from build123d import *

# Parameters (mm, degrees)
F0_W       = 2.5
F0_H       = 32
F0_H_2     = 52
F1_DEPTH   = 5
F2_DEPTH   = 20
F3_W       = 15
F3_H       = 15
F3_R       = 2.5
F4_W       = 15
F4_H       = 15
F4_R       = 2.5
F5_DEPTH   = 5
F6_SIZE2   = 2.14473742
F6_SIZE    = 2
F7_SIZE2   = 2.14473742
F7_SIZE    = 2
F8_SIZE2   = 2.14473742
F8_SIZE    = 2
F8_2_SIZE2 = 2.14473742
F8_2_SIZE  = 2


with BuildPart() as f1:
    # F0 (on Top) → F1 (new body)
    with BuildSketch(Plane.XY):
        Polygon((61.6508859247, 52.6726719439), (-55.3491140753, 52.6726719439), (-55.3491140753, 37.6726719439), (-52.8491140753, 37.6726719439), (-52.8491140753, 50.1726719439), (59.1508859247, 50.1726719439), (59.1508859247, 27.6726719439), (61.6508859247, 27.6726719439), align=None)
        Polygon((-52.8491140753, 50.1726719439), (-52.8491140753, 37.6726719439), (-52.8491140753, -14.3273280561), (-52.8491140753, -26.8273280561), (59.1508859247, -26.8273280561), (59.1508859247, -4.3273280561), (59.1508859247, 27.6726719439), (59.1508859247, 50.1726719439), align=None)
        with Locations((60.4008859247, 11.6726719439)):
            Rectangle(F0_W, F0_H)
        Polygon((-52.8491140753, -14.3273280561), (-55.3491140753, -14.3273280561), (-55.3491140753, -29.3273280561), (61.6508859247, -29.3273280561), (61.6508859247, -4.3273280561), (59.1508859247, -4.3273280561), (59.1508859247, -26.8273280561), (-52.8491140753, -26.8273280561), align=None)
        with Locations((-54.0991140753, 11.6726719439)):
            Rectangle(F0_W, F0_H_2)
    extrude(amount=-F1_DEPTH)

    # F0 (on Top) → F2 (join)
    with BuildSketch(Plane.XY):
        Polygon((61.6508859247, 52.6726719439), (-55.3491140753, 52.6726719439), (-55.3491140753, 37.6726719439), (-52.8491140753, 37.6726719439), (-52.8491140753, 50.1726719439), (59.1508859247, 50.1726719439), (59.1508859247, 27.6726719439), (61.6508859247, 27.6726719439), align=None)
        Polygon((-52.8491140753, -14.3273280561), (-55.3491140753, -14.3273280561), (-55.3491140753, -29.3273280561), (61.6508859247, -29.3273280561), (61.6508859247, -4.3273280561), (59.1508859247, -4.3273280561), (59.1508859247, -26.8273280561), (-52.8491140753, -26.8273280561), align=None)
    extrude(amount=F2_DEPTH)

    # F3 (on face) + F4 (on face) → F5 (join)
    with BuildSketch(Plane.XY.offset(20)):
        with Locations((-62.8491140753, 45.1726719439)):
            Rectangle(F3_W, F3_H)
        with Locations((-62.8491140753, 45.1726719439)):
            Circle(F3_R, mode=Mode.SUBTRACT)
        with Locations((69.1508859247, 45.1726719439)):
            Rectangle(F3_W, F3_H)
        with Locations((69.1508859247, 45.1726719439)):
            Circle(F3_R, mode=Mode.SUBTRACT)
    with BuildSketch(Plane.XY.offset(20)):
        with Locations((-62.8491140753, -21.8273280561)):
            Rectangle(F4_W, F4_H)
        with Locations((-62.8491140753, -21.8273280561)):
            Circle(F4_R, mode=Mode.SUBTRACT)
        with Locations((69.1508859247, -21.8273280561)):
            Rectangle(F4_W, F4_H)
        with Locations((69.1508859247, -21.8273280561)):
            Circle(F4_R, mode=Mode.SUBTRACT)
    extrude(amount=-F5_DEPTH)

    # F6
    f6_edges = [f1.edges().sort_by_distance(p)[0] for p in [
        (66.650886, -21.827328, 15),
    ]]
    f6_side = f1.faces().sort_by_distance((76.438754, -21.827328, 15))[0]
    chamfer(f6_edges, length=F6_SIZE, length2=F6_SIZE2, reference=f6_side)

    # F7
    f7_edges = [f1.edges().sort_by_distance(p)[0] for p in [
        (66.650886, 45.172672, 15),
    ]]
    f7_side = f1.faces().sort_by_distance((69.150886, 52.46054, 15))[0]
    chamfer(f7_edges, length=F7_SIZE, length2=F7_SIZE2, reference=f7_side)

    # F8
    f8_edges = [f1.edges().sort_by_distance(p)[0] for p in [
        (-65.349114, -21.827328, 15),
    ]]
    f8_side = f1.faces().sort_by_distance((-62.849114, -29.115196, 15))[0]
    chamfer(f8_edges, length=F8_SIZE, length2=F8_SIZE2, reference=f8_side)

    # F8#2
    f8_2_edges = [f1.edges().sort_by_distance(p)[0] for p in [
        (-65.349114, 45.172672, 15),
    ]]
    f8_2_side = f1.faces().sort_by_distance((-62.849114, 37.884804, 15))[0]
    chamfer(f8_2_edges, length=F8_2_SIZE, length2=F8_2_SIZE2, reference=f8_2_side)


solid = f1.part
Read the model definition and answer for the solid it produces. Units are mm, in the model's axes. A direction names the side the tool comes from. Coordinates: 2 decimals unless noted, no trailing zeros. Loops run counter-clockwise (first coordinate to the right, second up) from the corner with the lowest first, then second, coordinate; pieces in that order, holes last.
Q1. The part is cut by section B-B on x = -38. Write down the section's boundary in (y, z), and give its area (3 significant figures).
Q2. The part is cut by section A-A on z = 5. Write down the section's boundary in (x, y), and give its area (3 significant figures).
Q3. The mould has two halves that part along X. Classify faces 4 (the face through (2.8, 50.4, 20)), 5 (the face through (-70.349, -22, 18)), 6 (the face through (-52.849, 44, 10)), 7 (the face through (59.151, -15, 10)): +X half, -X half, draft (parallel to the pull), parting line (faces both ways), or undercut.
Q4. The part is cut by section C-C on y = -12. Write down the section's boundary in (x, z), and give its area (3 significant figures).
Q5. The part is cut by section D-D on z = -3. Write down the section's boundary in (x, y), and give its area (3 significant figures).
Q6. Each of these flat-tipped pins is pushed along its axis until it touches: pin 1 Ø6 at (y, z) = (-18.5, 5.5) entering from +X; pin 2 Ø4.5 at (x, y) = (-62.85, -21.83) entering from +Z; pin 3 Ø8 at (x, y) = (-62.85, 45.17) entering from -Z; pin 4 Ø10 at (y, z) = (35.5, 5.5) entering from -X. Where does it stop, or does it pass through?
Q7. Consider probe 1 along Y at (x, z) = (-4.5, 15.75); probe 2 along X at (y, z) = (4, -2.5); probe 3 along Z at (x, y) = (22, 19.5). Determine where each line is inside the solid, lowest interval first.
Q8. Which of the six approach directions +Z, -Z, +X, -X, +Y, -Y give full straight-line access (tool end or side, diameter ignored) to faces 1 (the face through (-52.849, -21, 10)), 2 (the face through (-66, 49, 15)), 3 (the face through (69, -14.327, 18))?
Results below:
1. outline: (-29.33, -5) - (52.67, -5) - (52.67, 20) - (50.17, 20) - (50.17, 0) - (-26.83, 0) - (-26.83, 20) - (-29.33, 20) - close
1. area: 510 mm2
2. outline: (-55.35, -29.33) - (61.65, -29.33) - (61.65, -4.33) - (59.15, -4.33) - (59.15, -26.83) - (-52.85, -26.83) - (-52.85, -14.33) - (-55.35, -14.33) - close; (-55.35, 37.67) - (-52.85, 37.67) - (-52.85, 50.17) - (59.15, 50.17) - (59.15, 27.67) - (61.65, 27.67) - (61.65, 52.67) - (-55.35, 52.67) - close
2. area: 760 mm2
3. face 4: draft
3. face 5: -X half
3. face 6: undercut
3. face 7: undercut
4. outline: (-55.35, -5) - (61.65, -5) - (61.65, 20) - (59.15, 20) - (59.15, 0) - (-55.35, 0) - close
4. area: 635 mm2
5. outline: (-55.35, -29.33) - (61.65, -29.33) - (61.65, 52.67) - (-55.35, 52.67) - close
5. area: 9,590 mm2
6. pin 1: stops at x = 61.65
6. pin 2: passes through
6. pin 3: stops at z = 15.53
6. pin 4: stops at x = -55.35
7. probe 1: y = -29.33 to -26.83, 50.17 to 52.67
7. probe 2: x = -55.35 to 61.65
7. probe 3: z = -5 to 0
8. face 1: +Z
8. face 2: -Z, -X, +Y, -Y
8. face 3: +Z, -Z, +X
